from build123d import *

# Parameters (mm, degrees)
BOSS_EXTRUDE1_DEPTH = 10


with BuildPart() as part:
    # Sketch1 → Boss-Extrude1 (new body)
    with BuildSketch(Plane(origin=(0, 0, 0), x_dir=(1, 0, 0), z_dir=(0, 1, 0))):
        Polygon((-135.812908411, 125.703692436), (-126.31291151, 125.703692436), (-126.31291151, 122.703686357), (-114.312909544, 122.703686357), (-114.312909544, 125.703692436), (-102.312915027, 125.703692436), (-102.312915027, 122.703686357), (-90.31291306, 122.703686357), (-90.31291306, 125.703692436), (-80.812908709, 125.703692436), (-80.812908709, 122.703686357), (-80.812908709, 118.703693151), (-83.812914789, 118.703693151), (-83.812914789, 106.703691185), (-80.812908709, 106.703691185), (-80.812908709, 94.703689218), (-83.812914789, 94.703689218), (-83.812914789, 82.703687251), (-80.812908709, 82.703687251), (-80.812908709, 75.703687966), (-135.812908411, 75.703687966), (-135.812908411, 82.703687251), (-132.812917233, 82.703687251), (-132.812917233, 94.703689218), (-135.812908411, 94.703689218), (-135.812908411, 106.703691185), (-132.812917233, 106.703691185), (-132.812917233, 118.703693151), (-135.812908411, 118.703693151), (-135.812908411, 122.703686357), align=None)
    extrude(amount=BOSS_EXTRUDE1_DEPTH)


solid = part.part
The model under review builds one solid part; all positions refer to its coordinate system, in mm. A direction names the side the tool comes from. Round coordinates to 2 decimals unless told otherwise and drop trailing zeros. Order: outer loops, then holes, each group sorted by start corner. A loop starts at its lowest first (then second) coordinate and runs counter-clockwise, first axis right, second up. Notation, with made-up numbers: (60, 69.5) -> (71, 69.5) arc R15 cw to (71, 73.5) -> close; hole circle Ø10 at (87.5, 36.25). An arc over 180 degrees is marked (long way). Return JSON: item names as keys, results as strings.
1. Take a section at C-C (z = -113). Write out the cut boundary in (x, y), then the cut area to 3 significant figures.
Answer block:
{"outline": "(-132.81, 0) -> (-83.81, 0) -> (-83.81, 10) -> (-132.81, 10) -> close", "area": "490 mm²"}
2. For faces 4 (the face through (-114.313, 5, -124)), 5 (the face through (-108, 10, -101)), 6 (the face through (-131, 5, -125.704)), 7 (the face through (-82, 5, -118.704)), 8 (the face through (-132.813, 5, -89)), list the 3-axis set-ups (+Z, -Z, +X, -X, +Y, -Y) from which the entire face can be reached by the end or side of a thin tool; tool diameter is ignored.
Answer block:
{"face 4": "-Z, +Y, -Y", "face 5": "+Z, -Z, +X, -X, +Y", "face 6": "-Z, +X, -X, +Y, -Y", "face 7": "+X, +Y, -Y", "face 8": "-X, +Y, -Y"}
3. Insertion check: P1, Ø3, axis at x = -97.5, y = 3.5, coming from the -Z side; P2, Ø3, axis at y = 6.5, z = -91, coming from the +X side; P3, Ø2, axis at y = 5, z = -114.5, coming from the -X side; P4, Ø6, axis at x = -92, z = -87, coming from the -Y side. Each pin has a flat end and moves straight along its axis. Give the tip position at first contact, or say it passes through.
Answer block:
{"P1": "stops at z = -122.7", "P2": "stops at x = -83.81", "P3": "stops at x = -132.81", "P4": "stops at y = 0"}
4. Take a section at A-A (y = 8). Write out the cut boundary in (x, z), then the cut area to 3 significant figures.
Answer block:
{"outline": "(-135.81, -125.7) -> (-126.31, -125.7) -> (-126.31, -122.7) -> (-114.31, -122.7) -> (-114.31, -125.7) -> (-102.31, -125.7) -> (-102.31, -122.7) -> (-90.31, -122.7) -> (-90.31, -125.7) -> (-80.81, -125.7) -> (-80.81, -118.7) -> (-83.81, -118.7) -> (-83.81, -106.7) -> (-80.81, -106.7) -> (-80.81, -94.7) -> (-83.81, -94.7) -> (-83.81, -82.7) -> (-80.81, -82.7) -> (-80.81, -75.7) -> (-135.81, -75.7) -> (-135.81, -82.7) -> (-132.81, -82.7) -> (-132.81, -94.7) -> (-135.81, -94.7) -> (-135.81, -106.7) -> (-132.81, -106.7) -> (-132.81, -118.7) -> (-135.81, -118.7) -> close", "area": "2,530 mm²"}
5. The part is to be moulded in two halves that separate along X. For faces 1 (the face through (-120, 5, -122.704)), 2 (the face through (-135.813, 5, -79)), 3 (the face through (-108, 0, -101)), say which applies: +X half, -X half, draft (parallel to the pull), parting line (faces both ways), or undercut.
Answer block:
{"face 1": "undercut", "face 2": "-X half", "face 3": "draft"}
6. Take a section at B-B (x = -94). Write out the cut boundary in (y, z).
Answer block:
{"outline": "(0, -122.7) -> (10, -122.7) -> (10, -75.7) -> (0, -75.7) -> close"}
7. For L1, parallel to Z at x = -133, y = 3.75; L2, parallel to X at y = 5, z = -113.5; L3, parallel to Z at x = -94, y = 0.5, list the stretches that pass through material, from the lowest coordinate up. Write a range as [from, to].
Answer block:
{"L1": "z = [-125.7, -118.7], [-106.7, -94.7], [-82.7, -75.7]", "L2": "x = [-132.81, -83.81]", "L3": "z = [-122.7, -75.7]"}
